Here's how the part is built. I have some questions about the finished solid (model axes, mm). A direction names the side the tool comes from. Give positions to 0.01 mm unless a question says otherwise; leave off trailing zeros. Loops run counter-clockwise (first coordinate to the right, second up) from the corner with the lowest first, then second, coordinate; pieces in that order, holes last.
Q1. I need wall thicknesses on probe 1 along X at (y, z) = (-2.5, 3); probe 2 along Y at (x, z) = (7, -2.25); probe 3 along Z at (x, y) = (0, 1). Which ranges of each line are inside material? Lowest first, please.
Q2. Suppose I cut it at A-A (x = 0). List the corners of the cut face in (y, z) for me.
Q3. Suppose I cut it at D-D (z = 10.25). Count the separate pieces of the cut face and the enclosed holes in it, and give its area (3 significant figures).
Q4. I'm going to push flat-ended pins straight in: P1, Ø6, axis at x = -4.5, z = 4, coming from the -Y side; P2, Ø3, axis at x = 4.24, z = 2.26, coming from the -Y side; P3, Ø4, axis at x = 4.5, y = -13.5, coming from the -Z side. Where does each tip first touch, or does it pass through?
Q5. Suppose I cut it at C-C (y = -14.5). List the corners of the cut face in (x, z) for me, and give its area (3 significant figures).
Q6. Thinking about a two-plate mould opening in Z: for faces 1 (the face through (-0.65, 0.99, 3.57)), 2 (the face through (0, -10, 0)), 3 (the face through (3.21, 1.34, 1.47)), 4 (the face through (0, -10, -1)), which applies, pulls with the +Z half, pulls with the -Z half, needs draft (parallel to the pull), parting line crosses it, or undercut?
Q7. For faces 5 (the face through (-2.6, 0, 4.2)), 6 (the face through (-0.2, -20, -0.5)), which set-ups out of +Z, -Z, +X, -X, +Y, -Y let a thin tool reach every point of the face, with its end or its side?
Q8. Suppose I cut it at B-B (z = 6.5). List the corners of the cut face in (x, y) for me, and give its area (3 significant figures).
```python
from build123d import *

# Parameters (mm, degrees)
F0_R           = 1.3
F0_R_2         = 3
F0_W           = 22
F0_H           = 4
F0_W_2         = 1
F0_H_2         = 4.5
F1_DEPTH       = 2
F2_DEPTH       = 20
F3_ANGLE       = 91
F4_D           = 2
F4_DEPTH       = 3
F4_CSINK_D     = 4
F4_CSINK_ANGLE = 90


with BuildPart() as f1:
    # F0 (on Front) → F1 (new body)
    with BuildSketch(Plane.XZ):
        with BuildLine():
            Line((10, 4.5), (11, 4.5))
            ThreePointArc((11, 4.5), (9.062743, 10.734316), (3.933329, 14.772727))
            ThreePointArc((3.933329, 14.772727), (0, 11.5), (-3.933329, 14.772727))
            ThreePointArc((-3.933329, 14.772727), (-9.062743, 10.734316), (-11, 4.5))
            Line((-11, 4.5), (-10, 4.5))
            Line((-10, 4.5), (-10, 0))
            Line((-10, 0), (10, 0))
            Line((10, 0), (10, 4.5))
        make_face()
        with Locations((-4.242641, 2.257359)):
            Circle(F0_R, mode=Mode.SUBTRACT)
        with Locations((4.242641, 2.257359)):
            Circle(F0_R, mode=Mode.SUBTRACT)
        with Locations((-4.242641, 10.742641)):
            Circle(F0_R, mode=Mode.SUBTRACT)
        with Locations((0, 6.5)):
            Circle(F0_R_2, mode=Mode.SUBTRACT)
        with Locations((4.242641, 10.742641)):
            Circle(F0_R, mode=Mode.SUBTRACT)
        with Locations((0, -3)):
            Rectangle(F0_W, F0_H)
        Polygon((-11, -1), (11, -1), (11, 0), (10, 0), (-10, 0), (-11, 0), align=None)
        with Locations((-10.5, 2.25)):
            Rectangle(F0_W_2, F0_H_2)
        with Locations((10.5, 2.25)):
            Rectangle(F0_W_2, F0_H_2)
    extrude(amount=-F1_DEPTH)



with BuildPart() as f2:
    # F0 (on Front) → F2 (new body)
    with BuildSketch(Plane.XZ):
        Polygon((-11, -1), (11, -1), (11, 0), (10, 0), (-10, 0), (-11, 0), align=None)
    extrude(amount=F2_DEPTH)


with BuildPart() as f1_1:
    add(f1.part)

    add(f2.part)  # F3 merges F2
    # F0 (on Front) → F3 (revolve)
    with BuildSketch(Plane.XZ):
        with Locations((-10.5, 2.25)):
            Rectangle(F0_W_2, F0_H_2)
        with Locations((10.5, 2.25)):
            Rectangle(F0_W_2, F0_H_2)
    revolve(axis=Axis((0, 0, 0), (1, 0, 0)), revolution_arc=F3_ANGLE)

    # F4
    with Locations(Plane.XZ):
        with Locations((-4.242641, 10.742641), (-4.242641, 2.257359), (4.242641, 2.257359), (4.242641, 10.742641)):
            CounterSinkHole(F4_D / 2, F4_CSINK_D / 2, depth=F4_DEPTH, counter_sink_angle=F4_CSINK_ANGLE)


solid = f1_1.part
```
Solutions:
1. probe 1: x = -11 to -10, 10 to 11
1. probe 2: y = 0 to 2
1. probe 3: z = -5 to 3.5, 9.5 to 11.5
2. outline: (-20, -1) - (0, -1) - (0, -5) - (2, -5) - (2, 3.5) - (0, 3.5) - (0, 0) - (-20, 0) - close; (0, 9.5) - (2, 9.5) - (2, 11.5) - (0, 11.5) - close
3. separate pieces: 3
3. enclosed holes: 0
3. area: 26.8 mm2
4. P1: stops at y = 0
4. P2: stops at y = 0.5
4. P3: stops at z = -1
5. outline: (-11, -1) - (11, -1) - (11, 0) - (-11, 0) - close
5. area: 22.0 mm2
6. face 1: undercut
6. face 2: pulls with the +Z half
6. face 3: undercut
6. face 4: pulls with the -Z half
7. face 5: +Z, -Y
7. face 6: +Z, -Z, +X, -X, -Y
8. outline: (-10.82, 0) - (-3, 0) - (-3, 2) - (-10.82, 2) - close; (3, 0) - (10.82, 0) - (10.82, 2) - (3, 2) - close
8. area: 31.3 mm2
